Autodesk Inventor part; units mm, degrees
ref_plane "YZ Plane" through (0, 0, 0) normal (1, 0, 0) x (0, 1, 0)
ref_plane "XZ Plane" through (0, 0, 0) normal (0, 1, 0) x (-1, 0, 0)
ref_plane "XY Plane" through (0, 0, 0) normal (0, 0, 1) x (1, 0, 0)
sketch "Sketch1" plane through (0, 0, 0) normal (0, 0, 1) x (1, 0, 0)
  circle A0 centre (0, 5) radius 1.5 construction
  circle A1 centre (0, -4.7587) radius 2.75 construction
  circle A2 centre (0, 5) radius 4
  line L0 (4, -7.5087) -> (-4, -7.5087)
  line L1 (-4, -7.5087) -> (-4, 5)
  line L2 (4, -7.5087) -> (4, 5)
  circle A3 centre (0, -4.7587) radius 2.85
  line L3 (2.85, -4.7587) -> (2.85, -7.5087)
  line L4 (-2.85, -4.7587) -> (-2.85, -7.5087)
  circle A4 centre (0, 5) radius 2
  point P0 (0, 0)
  dimension "d0" = 8
  dimension "d1" = 0.1
  dimension "d2" = 4
extrude "Extrusion1" add sketch "Sketch1" along normal blind 2 contours A2 | L2 L0 L3 A3 L4 L1 A2
sketch "Sketch3" plane through (0, 0, 2) normal (0, 0, 1) x (1, 0, 0)
  line L0 (-4, 5) -> (-4, -7.5087)
  line L1 (-4, -7.5087) -> (-2.85, -7.5087)
  line L2 (-2.85, -7.5087) -> (-2.85, -4.7587)
  arc A0 (2.85, -4.7587) -> (-2.85, -4.7587) centre (0, -4.7587) ccw
  line L3 (2.85, -4.7587) -> (2.85, -7.5087)
  line L4 (2.85, -7.5087) -> (4, -7.5087)
  line L5 (4, -7.5087) -> (4, 5)
  arc A1 (4, 5) -> (-4, 5) centre (0, 5) ccw
  circle A2 centre (0, 5) radius 2
  circle A3 centre (0, 5) radius 2 construction
  line L6 (0, 3) -> (0, -1.9087) construction
  line L7 (4, -7.5087) -> (4, 5)
  line L8 (4, 0.5456) -> (-4, 0.5456)
  arc A4 (2.85, -4.7587) -> (-2.85, -4.7587) centre (0, -4.7587) ccw
  point P0 (0, 0)
  point P1 (0, 0.5456)
  point P2 (0, -1.9087)
extrude "Extrusion2" add sketch "Sketch3" along normal blind 1 contours L8 L5 L4 L3 A0 L2 L1 L0
chamfer "Chamfer1" distance 1 angle 45 1 edges at (0, 0.5456, 3)
properties part number "display-retainer-tab"
CAD build for the part. Positions are in the model's coordinates, mm. A direction names the side the tool comes from. Round coordinates to 2 decimals unless told otherwise and drop trailing zeros. Loops run counter-clockwise (first coordinate to the right, second up) from the corner with the lowest first, then second, coordinate; pieces in that order, holes last.
(1) Which spindle directions (+Z, -Z, +X, -X, +Y, -Y) get a long thin tool onto all of the face, cutting with end or side? Do faces 4 (the cylindrical face through (0, 7, 1)), 5 (the flat face through (1, 3, 2)), 6 (the flat face through (-2.85, -6, 1)). Say none if no direction does.
(2) Cut at A-A (z = 0.65). Give the cut face in (x, y), plus the area to 3 significant figures.
(3) Drop flat-ended pins along their axis: pin 1 (2 mm diameter, centred on x = 1.5, y = 1, fed in from +Z); pin 2 (2.5 mm diameter, centred on x = 1, y = 4, fed in from +Z). Give the stop position or say it passes through.
(4) Wall check: line 1 along Y through (x, z) = (0, 1.25); line 2 along Z through (x, y) = (3.5, 2.5); line 3 along X through (y, z) = (-3.25, 1.8). Give the ranges that are in metal, low to high.
(5) Two-plate mould, pull along X, no slides. Class faces 1 (the flat face through (2.85, -6, 1)), 2 (the flat face through (4, -1, 1)), 3 (the cylindrical face through (0, 9, 1)): +X half, -X half, draft (parallel to the pull), parting line (faces both ways), or undercut.
(6) Cut at C-C (y = -2.5). Give the cut face in (x, z), plus the area to 3 significant figures.
Findings below:
1. face 4: +Z, -Z
1. face 5: +Z, +X, -X, +Y
1. face 6: +Z, -Z, -Y
2. outline: (-4, -7.51) - (-2.85, -7.51) - (-2.85, -4.76) arc R2.85 cw to (2.85, -4.76) - (2.85, -7.51) - (4, -7.51) - (4, 5) arc R4 ccw to (-4, 5) - close; hole circle Ø4 at (0, 5)
2. area: 84.2 mm2
3. pin 1: stops at z = 2.55
3. pin 2: stops at z = 2
4. line 1: y = -1.91 to 3, 7 to 9
4. line 2: z = 0 to 2
4. line 3: x = -4 to -2.42, 2.42 to 4
5. face 1: undercut
5. face 2: +X half
5. face 3: parting line
6. outline: (-4, 0) - (-1.74, 0) - (-1.74, 3) - (-4, 3) - close; (1.74, 0) - (4, 0) - (4, 3) - (1.74, 3) - close
6. area: 13.6 mm2
